Source: CAD feature listing. Evaluate the final solid. Frame: model axes, mm. Face numbers are marked on the shaded views. A direction names the side the tool comes from. Round coordinates to 2 decimals unless told otherwise and drop trailing zeros. Loops run counter-clockwise (first coordinate to the right, second up) from the corner with the lowest first, then second, coordinate; pieces in that order, holes last. Notation, with made-up numbers: M 31.25,47.25 L 76.25,47.25 A32 ccw 76.25,79.25 Z; hole C 17.5,22.25 d2. An arc over 180 degrees is marked long. Answer as a JSON object with one key per item and string values.
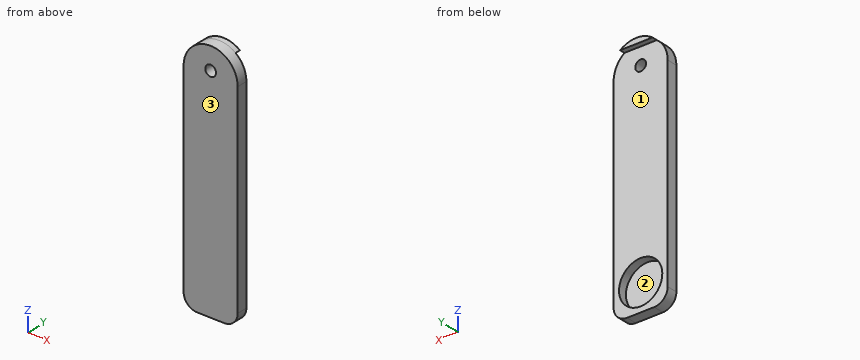
from build123d import *

# Parameters (mm, degrees)
SKETCH1_W           = 20
SKETCH1_H           = 80
BOSS_EXTRUDE1_DEPTH = 4
SKETCH8_R           = 10
BOSS_EXTRUDE2_DEPTH = 4
SKETCH9_R           = 8
CUT_EXTRUDE1_DEPTH  = 3.175
SKETCH10_R          = 2
CUT_EXTRUDE2_DEPTH  = 52.14684741
BOSS_EXTRUDE3_START = 2
BOSS_EXTRUDE3_DEPTH = 2
FILLET1_R           = 5


with BuildPart() as part:
    # Sketch1 → Boss-Extrude1 (new body)
    with BuildSketch(Plane(origin=(0, 0, 0), x_dir=(1, 0, 0), z_dir=(0, 1, 0))):
        Rectangle(SKETCH1_W, SKETCH1_H)
    extrude(amount=BOSS_EXTRUDE1_DEPTH)

    # Sketch8 → Boss-Extrude2 (add)
    with BuildSketch(Plane(origin=(0, 4, 0), x_dir=(1, 0, 0), z_dir=(0, 1, 0))):
        with Locations((0, -40)):
            Circle(SKETCH8_R)
    extrude(amount=-BOSS_EXTRUDE2_DEPTH)

    # Sketch9 → Cut-Extrude1 (cut)
    with BuildSketch(Plane(origin=(0, 4, 0), x_dir=(1, 0, 0), z_dir=(0, 1, 0))):
        with Locations(Location((0, 30, 0), (0, 0, 270))):
            Circle(SKETCH9_R)
    extrude(amount=-CUT_EXTRUDE1_DEPTH, mode=Mode.SUBTRACT)

    # Sketch10 → Cut-Extrude2 (cut, through all)
    with BuildSketch(Plane(origin=(0, 4, 0), x_dir=(1, 0, 0), z_dir=(0, 1, 0))):
        with Locations(Location((0, -41.7425, 0), (0, 0, 270))):
            Circle(SKETCH10_R)
    extrude(amount=-CUT_EXTRUDE2_DEPTH, mode=Mode.SUBTRACT)

    # Sketch11 → Boss-Extrude3 (add)
    with BuildSketch(Plane(origin=(0, 4, 0), x_dir=(1, 0, 0), z_dir=(0, 1, 0)).offset(BOSS_EXTRUDE3_START)):
        with BuildLine():
            Line((-6, -48), (6, -48))
            ThreePointArc((6, -48), (0, -50), (-6, -48))
        make_face()
    extrude(amount=-BOSS_EXTRUDE3_DEPTH)

    # Fillet1
    fillet1_edges = [part.edges().sort_by_distance(p)[0] for p in [
        (-10, 2, -40),
        (10, 2, -40),
    ]]
    fillet(fillet1_edges, radius=FILLET1_R)


solid = part.part
Item 1: Section B-B on z = -30. Return the cut outline in (x, y) (3 decimals), then the cut area to 3 significant figures.
Answer sheet:
{"outline": "M -10,0 L 10,0 L 10,4 L 8,4 L 8,0.825 L -8,0.825 L -8,4 L -10,4 Z", "area": "29.2 mm²"}
Item 2: Access query for the marked faces 1, 2 and 3. Directions: +Z, -Z, +X, -X, +Y, -Y. A direction counts if a zero-diameter tool reaches every point of the face in a straight line with its end or side. Return the directions, or none.
Answer sheet:
{"face 1": "-Z, +X, -X, +Y", "face 2": "+Y", "face 3": "+Z, -Z, +X, -X, -Y"}
Item 3: Section C-C on y = 3.25. Return the cut outline in (x, z), then the cut area to 3 significant figures.
Answer sheet:
{"outline": "M -10,-35 A5 ccw -5,-40 L 5,-40 A5 ccw 10,-35 L 10,40 A10 ccw -10,40 Z; hole C 0,-30 d16; hole C 0,41.74 d4", "area": "1,530 mm²"}
Item 4: Section D-D on z = -10. Return the cut outline in (x, y), then the cut area to 3 significant figures.
Answer sheet:
{"outline": "M -10,0 L 10,0 L 10,4 L -10,4 Z", "area": "80.0 mm²"}
Item 5: Line query: probe 1 along Z at (x, y) = (-0.25, 2.1); probe 2 along X at (y, z) = (1, -30.5); probe 3 along Y at (x, z) = (-5.5, 7). Output: solid intervals per line, ascending. Write a range as from..to.
Answer sheet:
{"probe 1": "z = -40..-38, -22..39.76, 43.73..50", "probe 2": "x = -10..-7.98, 7.98..10", "probe 3": "y = 0..4"}
Item 6: Section A-A on x = 0. Return the cut outline in (y, z) (1 decimal).
Answer sheet:
{"outline": "M 0,-40 L 4,-40 L 4,-38 L 0.8,-38 L 0.8,-22 L 4,-22 L 4,39.7 L 0,39.7 Z; M 0,43.7 L 4,43.7 L 4,48 L 6,48 L 6,50 L 0,50 Z"}
Item 7: Contact query for flat-ended pins moving along their axis: pin 1 Ø2 at (x, y) = (0.5, 5.5) entering from -Z; pin 2 Ø10 at (x, z) = (4, -10) entering from +Y. Output: stop coordinate, or through.
Answer sheet:
{"pin 1": "stops at z = 48", "pin 2": "stops at y = 4"}
